from build123d import *

# Parameters (mm, degrees)
F0_W     = 70.202325
F0_H     = 77.687127
F0_W_2   = 41.811679
F0_H_2   = 39.230711
F1_DEPTH = 50.8
F2_W     = 31.745904
F2_H     = 30.455421
F3_DEPTH = 25.4


with BuildPart() as f1:
    # F0 (on Front) → F1 (new body)
    with BuildSketch(Plane.XZ):
        with Locations((-16.518192, 17.937724)):
            Rectangle(F0_W, F0_H)
        with Locations((-27.100162, 8.001)):
            Rectangle(F0_W_2, F0_H_2, mode=Mode.SUBTRACT)
        with Locations((-27.100162, 8.001)):
            Rectangle(F0_W_2, F0_H_2)
    extrude(amount=-F1_DEPTH)

    # F2 (on face) → F3 (join)
    with BuildSketch(Plane.XZ):
        with Locations((-29.035888, 12.130549)):
            Rectangle(F2_W, F2_H)
    extrude(amount=F3_DEPTH)


solid = f1.part
Design review of the part built by this model. Coordinates are the model's own, in mm. A direction names the side the tool comes from. Coordinates: 2 decimals unless noted, no trailing zeros. Loops run counter-clockwise (first coordinate to the right, second up) from the corner with the lowest first, then second, coordinate; pieces in that order, holes last.
Item 1: Clearance check with flat-ended pins moving along their axes: pin 1 (10 mm diameter, centred on y = -17.5, z = 18, fed in from -X); pin 2 (1.5 mm diameter, centred on x = -22, z = 47, fed in from -Y); pin 3 (12 mm diameter, centred on y = -5.5, z = 33, fed in from +X); pin 4 (7.5 mm diameter, centred on y = -16, z = 8, fed in from +X). State where each tip first meets the part, or that it passes through.
Completed:
pin 1: stops at x = -44.91
pin 2: stops at y = 0
pin 3: stops at x = 18.58
pin 4: stops at x = -13.16
Item 2: Add section D-D (z = -9.5). Write out the cut boundary in (x, y), and give its area (3 significant figures).
Completed:
outline: (-51.62, 0) - (18.58, 0) - (18.58, 50.8) - (-51.62, 50.8) - close
area: 3,570 mm2
Item 3: Add section B-B (z = 3). Write out the cut boundary in (x, y), and give its area (3 significant figures).
Completed:
outline: (-51.62, 0) - (-44.91, 0) - (-44.91, -25.4) - (-13.16, -25.4) - (-13.16, 0) - (18.58, 0) - (18.58, 50.8) - (-51.62, 50.8) - close
area: 4,370 mm2
Item 4: Wall thickness on L1, parallel to Y at x = -11, z = -7; L2, parallel to X at y = -5, z = 21; L3, parallel to Z at x = -36, y = -1: over which ranges is each line inside the solid? List them lowest first.
Completed:
L1: y = 0 to 50.8
L2: x = -44.91 to -13.16
L3: z = -3.1 to 27.36
Item 5: For faces 1 (the flat face through (-13.163, -13, 12)), 2 (the flat face through (-29, -13, 27.358)), 3 (the flat face through (18.583, 25, 17)), 4 (the flat face through (-44.909, -13, 12)), 5 (the flat face through (-29, -13, -3.097)), list the 3-axis set-ups (+Z, -Z, +X, -X, +Y, -Y) from which the entire face can be reached by the end or side of a thin tool; tool diameter is ignored.
Completed:
face 1: +Z, -Z, +X, -Y
face 2: +Z, +X, -X, -Y
face 3: +Z, -Z, +X, +Y, -Y
face 4: +Z, -Z, -X, -Y
face 5: -Z, +X, -X, -Y
Item 6: Add section A-A (x = -30.5). Write out the cut boundary in (y, z).
Completed:
outline: (-25.4, -3.1) - (0, -3.1) - (0, -20.91) - (50.8, -20.91) - (50.8, 56.78) - (0, 56.78) - (0, 27.36) - (-25.4, 27.36) - close
Item 7: Add section C-C (y = -5). Write out the cut boundary in (x, z), and give its area (3 significant figures).
Completed:
outline: (-44.91, -3.1) - (-13.16, -3.1) - (-13.16, 27.36) - (-44.91, 27.36) - close
area: 967 mm2
